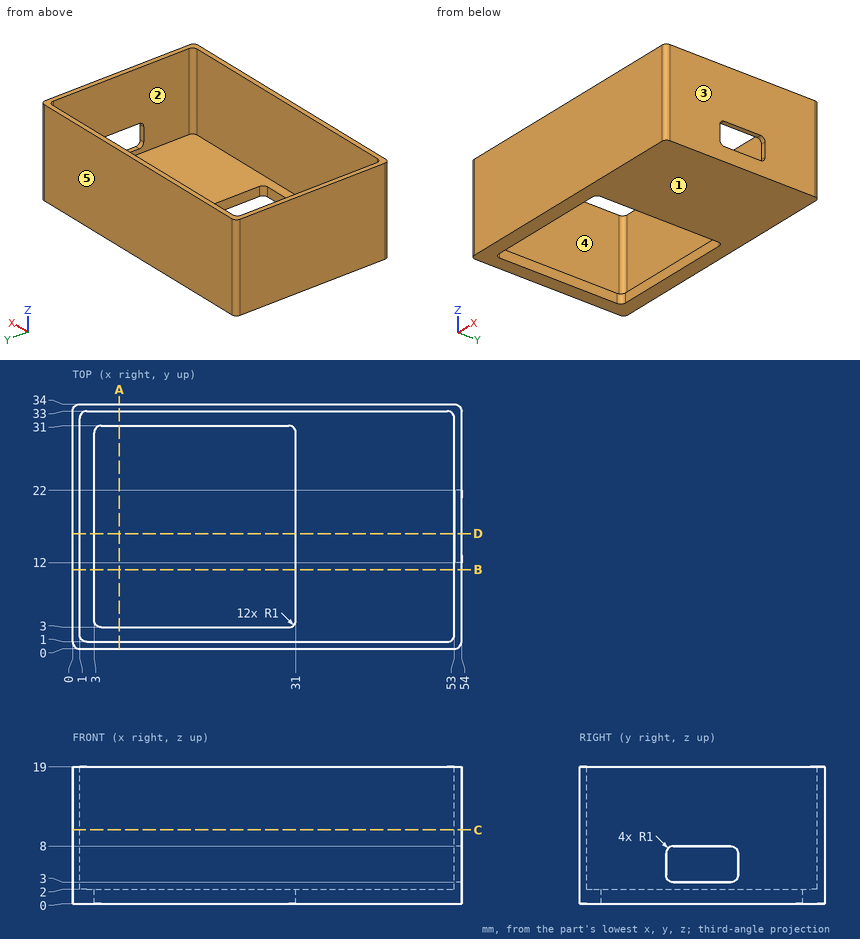
Print and shaded views of the part. All mm, measured from the part's lowest x, y and z. A direction names the side the tool comes from. Coordinates: 2 decimals unless noted, no trailing zeros. Loops run counter-clockwise (first coordinate to the right, second up) from the corner with the lowest first, then second, coordinate; pieces in that order, holes last. Notation, with made-up numbers: (73, 81) - (77, 81) arc R13 cw to (77, 89) - close; hole circle Ø4 at (84.5, -24.5). An arc over 180 degrees is marked (long way). Write item = value, one per line. Start each with the question number.
Item 1: 3-axis set-ups, long thin cutter, end or side, ignore diameter. For the marked faces 1 and 2: which of +Z, -Z, +X, -X, +Y, -Y reach the whole face in a straight line?
Item 2: Flat gauge pins, fed straight in: pin 1 Ø1.1 at (x, z) = (53.5, 6) entering from +Y; pin 2 Ø9.5 at (x, y) = (39, 21.5) entering from +Z; pin 3 Ø0.5 at (x, z) = (53.5, 6) entering from -Y. Where does each tip first touch, or does it go through?
Item 3: Cut at A-A, the plane x = 6.5. Give the cut face in (y, z).
Item 4: Mould opens along Y. For the marked faces 3, 4 and 5 say: released by +Y, released by -Y, zero draft, split by the parting line, or undercut.
Item 5: Cut at D-D, the plane y = 16. Give the cut face in (x, z), and give its area (3 significant figures).
Item 6: Cut at B-B, the plane y = 11. Give the cut face in (x, z).
Item 7: Wall check: L1, parallel to Y at x = 26, z = 9.5; L2, parallel to X at y = 29, z = 4; L3, parallel to Z at x = 40.5, y = 32. Give the ranges that are in metal, low to high. Write a range as from..to.
Item 8: Cut at C-C, the plane z = 10.25. Give the cut face in (x, y).
The answers:
q1.face_1 = -Z, +X, -X, +Y, -Y
q1.face_2 = +Z
q2.pin_1 = 34
q2.pin_2 = 2
q2.pin_3 = 0.03
q3.outline = (0, 0) - (3, 0) - (3, 2) - (1, 2) - (1, 19) - (0, 19) - close; (31, 0) - (34, 0) - (34, 19) - (33, 19) - (33, 2) - (31, 2) - close
q4.face_3 = zero draft
q4.face_4 = undercut
q4.face_5 = released by +Y
q5.outline = (0, 0) - (3, 0) - (3, 2) - (1, 2) - (1, 19) - (0, 19) - close; (31, 0) - (54, 0) - (54, 3) - (53, 3) - (53, 2) - (31, 2) - close; (53, 8) - (54, 8) - (54, 19) - (53, 19) - close
q5.area = 81.0 mm2
q6.outline = (0, 0) - (3, 0) - (3, 2) - (1, 2) - (1, 19) - (0, 19) - close; (31, 0) - (54, 0) - (54, 19) - (53, 19) - (53, 2) - (31, 2) - close
q7.L1 = 0..1, 33..34
q7.L2 = 0..1, 53..54
q7.L3 = 0..2
q8.outline = (0, 1) arc R1 ccw to (1, 0) - (53, 0) arc R1 ccw to (54, 1) - (54, 33) arc R1 ccw to (53, 34) - (1, 34) arc R1 ccw to (0, 33) - close; hole (1, 2) arc R1 ccw to (2, 1) - (52, 1) arc R1 ccw to (53, 2) - (53, 32) arc R1 ccw to (52, 33) - (2, 33) arc R1 ccw to (1, 32) - close
